Geometry check sheet. Reference: the model listing, model coordinates, mm. A direction names the side the tool comes from. Coordinates: 2 decimals unless noted, no trailing zeros. Order: outer loops, then holes, each group sorted by start corner. A loop starts at its lowest first (then second) coordinate and runs counter-clockwise, first axis right, second up. Notation, with made-up numbers: M 22,85.5 L 59,85.5 A25 ccw 59,105.5 Z; hole C 33,-33.75 d5. An arc over 180 degrees is marked long. One line per item, written item: value. Start each with the question number.
1) Sectioned sample at C-C, the plane z = 6.25. Enter the section's corners in (x, y), then the cut area to 3 significant figures.
2) Draft check along Z on faces 1 (the flat face through (-0.411, 9.453, 5.916)), 2 (the flat face through (-1, 7, 0)), 3 (the cylindrical face through (-1.17, 6.09, 4.78)). Enter one of: pulls with the +Z half, pulls with the -Z half, needs draft (parallel to the pull), parting line crosses it, or undercut.
3) Sectioned sample at B-B, the plane x = -2.75. Enter the section's corners in (y, z), then the cut area to 3 significant figures.
4) Thickness scan on L1, parallel to Z at x = -1.75, y = 5.25; L2, parallel to Z at x = -1.75, y = 7.75; L3, parallel to X at y = 4.75, z = 3. Record the ranges inside material, lowest first. Write a range as from..to.
5) Access from +Z, -Z, +X, -X, +Y, -Y to the whole of each face (thin tool, end or side, straight path). Record for faces 4 (the flat face through (-1.28, 8.63, 6.02)), 5 (the flat face through (-2.292, 9.187, 5.916)).
6) Go/stop test with flat-tipped pins: P1, Ø2, axis at y = 6, z = 3, coming from the +X side; P2, Ø1, axis at y = 7, z = 9, coming from the +X side; P3, Ø1.5, axis at x = -1.5, z = 1, coming from the -Y side; P4, Ø2, axis at y = 9, z = 6, coming from the -X side. Record where each tip stops, or that it passes through.
7) Sectioned sample at A-A, the plane z = 8. Enter the section's corners in (x, y), then the cut area to 3 significant figures.
```python
from build123d import *

# Parameters (mm, degrees)
F1_DEPTH = 12
F2_R     = 1.25
F3_DEPTH = 5


with BuildPart() as f1:
    # F0 (on Top) → F1 (new body)
    with BuildSketch(Plane.XY):
        with BuildLine():
            Line((-0.5398019886, 3.6867167497), (-1.340078938, 9.1524143503))
            ThreePointArc((-1.340078938, 9.1524143503), (-2.2779450693, 8.9651249998), (-3.19145978, 8.6819977236))
            Line((-3.19145978, 8.6819977236), (-2.4197573686, 3.4114572922))
            Line((-2.4197573686, 3.4114572922), (-0.5398019886, 3.6867167497))
        make_face()
        with BuildLine():
            Line((1.3401533915, 3.9619762073), (0.5684509802, 9.2325166387))
            ThreePointArc((0.5684509802, 9.2325166387), (-0.3878872523, 9.2418636367), (-1.340078938, 9.1524143503))
            Line((-1.340078938, 9.1524143503), (-0.5398019886, 3.6867167497))
            Line((-0.5398019886, 3.6867167497), (1.3401533915, 3.9619762073))
        make_face()
        with BuildLine():
            ThreePointArc((-1.340078938, 9.1524143503), (-0.3878872523, 9.2418636367), (0.5684509802, 9.2325166387))
            Line((0.5684509802, 9.2325166387), (0.5603502186, 9.2878428764))
            Line((0.5603502186, 9.2878428764), (-1.4090423808, 9.6234179499))
            Line((-1.4090423808, 9.6234179499), (-1.340078938, 9.1524143503))
        make_face()
        with BuildLine():
            ThreePointArc((-3.19145978, 8.6819977236), (-2.2779450693, 8.9651249998), (-1.340078938, 9.1524143503))
            Line((-1.340078938, 9.1524143503), (-1.4090423808, 9.6234179499))
            Line((-1.4090423808, 9.6234179499), (-3.1995605415, 8.7373239614))
            Line((-3.1995605415, 8.7373239614), (-3.19145978, 8.6819977236))
        make_face()
    extrude(amount=F1_DEPTH)

    # F2 (on face) → F3 (cut)
    with BuildSketch(Plane(origin=(-0.5398019886, 3.6867167497, 0), x_dir=(0.9894502, 0.1448733987, 0), z_dir=(0.1448733987, -0.9894502, 0))):
        with Locations((0, 6)):
            Circle(F2_R)
    extrude(amount=-F3_DEPTH, mode=Mode.SUBTRACT)


solid = f1.part
```
Final values:
1. outline: M -3.2,8.74 L -2.42,3.41 L -1.75,3.51 L -2.48,8.46 L -0.05,8.81 L 0.67,3.86 L 1.34,3.96 L 0.56,9.29 L -1.41,9.62 Z
1. area: 9.38 mm^2
2. face 1: needs draft
2. face 2: pulls with the -Z half
2. face 3: undercut
3. outline: M 5.67,0 L 8.96,0 L 8.96,12 L 5.67,12 Z
3. area: 39.5 mm^2
4. L1: z = 0..5.21, 6.79..12
4. L2: z = 0..4.91, 7.09..12
4. L3: x = -2.62..1.22
5. face 4: none
5. face 5: +Z, -Z, -X, +Y
6. P1: stops at x = 1.19
6. P2: stops at x = 0.97
6. P3: stops at y = 3.44
6. P4: stops at x = -3.2
7. outline: M -3.2,8.74 L -2.42,3.41 L 1.34,3.96 L 0.56,9.29 L -1.41,9.62 Z
7. area: 21.6 mm^2
